Geometry check sheet. Reference: the model listing, model coordinates, mm. A direction names the side the tool comes from. Coordinates: 2 decimals unless noted, no trailing zeros. Loops run counter-clockwise (first coordinate to the right, second up) from the corner with the lowest first, then second, coordinate; pieces in that order, holes last.
from build123d import *

# Parameters (mm, degrees)
F1_DEPTH = 20.955
F2_DEPTH = 6.35


with BuildPart() as f1:
    # F0 (on Front) → F1 (new body)
    with BuildSketch(Plane.XZ):
        Polygon((0, 418.380344), (1745.243721, 0), (1854.2, 0), (0, 444.5), align=None)
        Polygon((0, 444.5), (1854.2, 0), (1854.2, 26.119656), (108.956279, 444.5), align=None)
    extrude(amount=F1_DEPTH)

    # F0 (on Front) → F2 (join)
    with BuildSketch(Plane.XZ):
        Polygon((0, 392.260688), (1636.287443, 0), (1745.243721, 0), (0, 418.380344), align=None)
        Polygon((0, 418.380344), (1745.243721, 0), (1854.2, 0), (0, 444.5), align=None)
        Polygon((0, 444.5), (1854.2, 0), (1854.2, 26.119656), (108.956279, 444.5), align=None)
        Polygon((108.956279, 444.5), (1854.2, 26.119656), (1854.2, 52.239312), (217.912557, 444.5), align=None)
    extrude(amount=F2_DEPTH)


solid = f1.part
(1) Gauge pin test, flat ends, axial feed: pin 1 Ø1 at (x, y) = (963.5, -13) entering from +Z; pin 2 Ø12 at (x, y) = (1594, -13.5) entering from +Z; pin 3 Ø3 at (x, y) = (1300.5, -10.5) entering from +Z; pin 4 Ø12 at (x, z) = (550, 254) entering from -Y. Record the tip position at first contact, or that the pin passes through.
Findings:
pin 1: stops at z = 239.76
pin 2: stops at z = 89.93
pin 3: stops at z = 159.22
pin 4: passes through
(2) Sectioned sample at C-C on z = 98.5. Record the cut outline in (x, y) (3 decimals).
Findings:
outline: (1225.402, -6.35) - (1334.358, -6.35) - (1334.358, -20.955) - (1552.271, -20.955) - (1552.271, -6.35) - (1661.227, -6.35) - (1661.227, 0) - (1225.402, 0) - close
(3) Access from +Z, -Z, +X, -X, +Y, -Y to the whole of each face (thin tool, end or side, straight path). Record for faces 1 (the flat face through (1047.51, -3.131, 245.624)), 2 (the flat face through (1042, -6.35, 236)), 3 (the flat face through (860.405, -13.55, 212.119)).
Findings:
face 1: +Z, +X, +Y, -Y
face 2: +Z, +X, -Y
face 3: -Z, -X, -Y
(4) Sectioned sample at B-B on x = 1719.5. Record the cut outline in (y, z) (3 decimals), and give its area (3 significant figures).
Findings:
outline: (-20.955, 6.171) - (-6.35, 6.171) - (-6.35, 0) - (0, 0) - (0, 84.53) - (-6.35, 84.53) - (-6.35, 58.411) - (-20.955, 58.411) - close
area: 1,300 mm2
(5) Scan lines: L1, parallel to Z at x = 185, y = -11.5; L2, parallel to Z at x = 218, y = -11.75; L3, parallel to Y at x = 844.5, z = 191.5. Record each from-to range of solid material in increasing order.
Findings:
L1: z = 374.03 to 426.27
L2: z = 366.12 to 418.36
L3: y = -6.35 to 0
(6) Sectioned sample at A-A on y = -13.75. Record the cut outline in (x, z), and give its area (3 significant figures).
Findings:
outline: (0, 418.38) - (1745.24, 0) - (1854.2, 0) - (1854.2, 26.12) - (108.96, 444.5) - (0, 444.5) - close
area: 94,000 mm2
